from build123d import *

# Parameters (mm, degrees)
SKETCH_1_W          = 125.6
SKETCH_1_H          = 165
SKETCH_1_R          = 2
SKETCH_1_R_2        = 12.5
SKETCH_1_R_3        = 2.25
SKETCH_1_R_4        = 1.5
SKETCH_1_W_2        = 10
SKETCH_1_H_2        = 23
SKETCH_1_W_3        = 16
SKETCH_1_H_3        = 40
EXTRUDE_1_DEPTH     = 1.5
SKETCH_2_W          = 1.2
SKETCH_2_H          = 100
SKETCH_2_H_2        = 50
EXTRUDE_2_DEPTH     = 45
SKETCH_3_W          = 125.6
SKETCH_3_H          = 1.2
SKETCH_3_W_2        = 22.4
EXTRUDE_3_DEPTH     = 5
SKETCH_4_W          = 22.4
SKETCH_4_H          = 3
SKETCH_4_W_2        = 125.6
EXTRUDE_4_DEPTH     = 1
SKETCH_5_W          = 125.6
SKETCH_5_H          = 3
EXTRUDE_5_DEPTH     = 1
FILLET_1_R          = 40
SKETCH_6_R          = 1.5
EXTRUDE_6_DEPTH     = 2
EXTRUDE_7_DEPTH     = 30
CUT_EXTRUDE_1_REACH = 214.515
SKETCH_9_R          = 1.5
SKETCH_10_R         = 1.5
CUT_EXTRUDE_2_DEPTH = 213.514964179
SKETCH_11_R         = 1.5
CUT_EXTRUDE_3_DEPTH = 213.514964179


with BuildPart() as part:
    # 草图1 → 凸台-拉伸1 (new body)
    with BuildSketch(Plane(origin=(0, 0, 0), x_dir=(1, 0, 0), z_dir=(0, 1, 0))):
        with Locations((62.8, 82.5)):
            Rectangle(SKETCH_1_W, SKETCH_1_H)
        with Locations(Location((93.2, 30, 0), (0, 0, 270))):
            Circle(SKETCH_1_R, mode=Mode.SUBTRACT)
        with Locations(Location((93.2, 88, 0), (0, 0, 270))):
            Circle(SKETCH_1_R, mode=Mode.SUBTRACT)
        with Locations(Location((7.2, 30, 0), (0, 0, 90))):
            Circle(SKETCH_1_R, mode=Mode.SUBTRACT)
        with Locations(Location((7.2, 88, 0), (0, 0, 90))):
            Circle(SKETCH_1_R, mode=Mode.SUBTRACT)
        with Locations(Location((33.8, 135, 0), (0, 0, 270))):
            Circle(SKETCH_1_R_2, mode=Mode.SUBTRACT)
        with Locations(Location((91.8, 135, 0), (0, 0, 90))):
            Circle(SKETCH_1_R_2, mode=Mode.SUBTRACT)
        with Locations(Location((49.3, 150.5, 0), (0, 0, 270))):
            Circle(SKETCH_1_R_3, mode=Mode.SUBTRACT)
        with Locations(Location((18.3, 150.5, 0), (0, 0, 90))):
            Circle(SKETCH_1_R_3, mode=Mode.SUBTRACT)
        with Locations(Location((49.3, 119.5, 0), (0, 0, 90))):
            Circle(SKETCH_1_R_3, mode=Mode.SUBTRACT)
        with Locations(Location((18.3, 119.5, 0), (0, 0, 270))):
            Circle(SKETCH_1_R_3, mode=Mode.SUBTRACT)
        with Locations(Location((107.3, 119.5, 0), (0, 0, 90))):
            Circle(SKETCH_1_R_3, mode=Mode.SUBTRACT)
        with Locations(Location((76.3, 119.5, 0), (0, 0, 270))):
            Circle(SKETCH_1_R_3, mode=Mode.SUBTRACT)
        with Locations(Location((107.3, 150.5, 0), (0, 0, 270))):
            Circle(SKETCH_1_R_3, mode=Mode.SUBTRACT)
        with Locations(Location((76.3, 150.5, 0), (0, 0, 90))):
            Circle(SKETCH_1_R_3, mode=Mode.SUBTRACT)
        with Locations(Location((122.1, 161, 0), (0, 0, 270))):
            Circle(SKETCH_1_R_4, mode=Mode.SUBTRACT)
        with Locations(Location((122.1, 109, 0), (0, 0, 90))):
            Circle(SKETCH_1_R_4, mode=Mode.SUBTRACT)
        with Locations(Location((109.1, 109, 0), (0, 0, 270))):
            Circle(SKETCH_1_R_4, mode=Mode.SUBTRACT)
        with Locations(Location((109.1, 161, 0), (0, 0, 90))):
            Circle(SKETCH_1_R_4, mode=Mode.SUBTRACT)
        with Locations(Location((16.5, 109, 0), (0, 0, 90))):
            Circle(SKETCH_1_R_4, mode=Mode.SUBTRACT)
        with Locations(Location((3.5, 109, 0), (0, 0, 270))):
            Circle(SKETCH_1_R_4, mode=Mode.SUBTRACT)
        with Locations(Location((16.5, 161, 0), (0, 0, 270))):
            Circle(SKETCH_1_R_4, mode=Mode.SUBTRACT)
        with Locations(Location((3.5, 161, 0), (0, 0, 90))):
            Circle(SKETCH_1_R_4, mode=Mode.SUBTRACT)
        with Locations(Location((69.1, 109, 0), (0, 0, 270))):
            Circle(SKETCH_1_R_4, mode=Mode.SUBTRACT)
        with Locations(Location((82.1, 109, 0), (0, 0, 90))):
            Circle(SKETCH_1_R_4, mode=Mode.SUBTRACT)
        with Locations(Location((82.1, 161, 0), (0, 0, 270))):
            Circle(SKETCH_1_R_4, mode=Mode.SUBTRACT)
        with Locations(Location((69.1, 161, 0), (0, 0, 90))):
            Circle(SKETCH_1_R_4, mode=Mode.SUBTRACT)
        with Locations(Location((56.5, 161, 0), (0, 0, 270))):
            Circle(SKETCH_1_R_4, mode=Mode.SUBTRACT)
        with Locations(Location((43.5, 161, 0), (0, 0, 90))):
            Circle(SKETCH_1_R_4, mode=Mode.SUBTRACT)
        with Locations(Location((56.5, 109, 0), (0, 0, 90))):
            Circle(SKETCH_1_R_4, mode=Mode.SUBTRACT)
        with Locations(Location((43.5, 109, 0), (0, 0, 270))):
            Circle(SKETCH_1_R_4, mode=Mode.SUBTRACT)
        with Locations(Location((4, 100, 0), (0, 0, 270))):
            Circle(SKETCH_1_R_4, mode=Mode.SUBTRACT)
        with Locations(Location((4, 6, 0), (0, 0, 270))):
            Circle(SKETCH_1_R_4, mode=Mode.SUBTRACT)
        with Locations(Location((121.6, 6, 0), (0, 0, 90))):
            Circle(SKETCH_1_R_4, mode=Mode.SUBTRACT)
        with Locations(Location((121.6, 100, 0), (0, 0, 90))):
            Circle(SKETCH_1_R_4, mode=Mode.SUBTRACT)
        with Locations((114.4, 66.5)):
            Rectangle(SKETCH_1_W_2, SKETCH_1_H_2, mode=Mode.SUBTRACT)
        with Locations((62.8, 135)):
            Rectangle(SKETCH_1_W_3, SKETCH_1_H_3, mode=Mode.SUBTRACT)
    extrude(amount=EXTRUDE_1_DEPTH)

    # 草图2 → 凸台-拉伸2 (add)
    with BuildSketch(Plane(origin=(0, 1.5, 0), x_dir=(1, 0, 0), z_dir=(0, 1, 0))):
        with Locations((0.6, 50)):
            Rectangle(SKETCH_2_W, SKETCH_2_H)
        with Locations((103.8, 25)):
            Rectangle(SKETCH_2_W, SKETCH_2_H_2)
        with Locations((125, 50)):
            Rectangle(SKETCH_2_W, SKETCH_2_H)
    extrude(amount=EXTRUDE_2_DEPTH)

    # 草图3 → 凸台-拉伸3 (add)
    with BuildSketch(Plane(origin=(0, 1.5, 0), x_dir=(1, 0, 0), z_dir=(0, 1, 0))):
        with Locations((62.8, 0.6)):
            Rectangle(SKETCH_3_W, SKETCH_3_H)
        with Locations((62.8, 99.4)):
            Rectangle(SKETCH_3_W, SKETCH_3_H)
        with Locations((114.4, 47.8)):
            Rectangle(SKETCH_3_W_2, SKETCH_3_H)
    extrude(amount=EXTRUDE_3_DEPTH)

    # 草图4 → 凸台-拉伸4 (add)
    with BuildSketch(Plane.XY):
        with Locations((114.4, 23.5)):
            Rectangle(SKETCH_4_W, SKETCH_4_H)
        with Locations((62.8, 44.7)):
            Rectangle(SKETCH_4_W_2, SKETCH_4_H)
    extrude(amount=-EXTRUDE_4_DEPTH)

    # 草图5 → 凸台-拉伸5 (add)
    with BuildSketch(Plane(origin=(0, 0, -100), x_dir=(-1, 0, 0), z_dir=(0, 0, -1))):
        with Locations((-62.8, 44.7)):
            Rectangle(SKETCH_5_W, SKETCH_5_H)
    extrude(amount=-EXTRUDE_5_DEPTH)

    # 圆角1
    fillet_1_edges = [part.edges().sort_by_distance(p)[0] for p in [
        (103.8, 46.5, -50),
    ]]
    fillet(fillet_1_edges, radius=FILLET_1_R)

    # 草图6 → 凸台-拉伸6 (add)
    # profile 1 of 4: a face of its own
    with BuildSketch(Plane(origin=(0, 46.5, 0), x_dir=(1, 0, 0), z_dir=(0, 1, 0))):
        with BuildLine():
            Line((0, 0), (10, 0))
            Line((10, 0), (10, 7))
            ThreePointArc((10, 7), (9.121320344, 9.121320344), (7, 10))
            Line((7, 10), (0, 10))
            Line((0, 10), (0, 0))
        make_face()
        with Locations(Location((5, 5, 0), (0, 0, 270))):
            Circle(SKETCH_6_R, mode=Mode.SUBTRACT)
    # profile 2 of 4: a face of its own
    with BuildSketch(Plane(origin=(0, 46.5, 0), x_dir=(1, 0, 0), z_dir=(0, 1, 0))):
        with BuildLine():
            Line((10, 100), (10, 93))
            ThreePointArc((10, 93), (9.121320344, 90.878679656), (7, 90))
            Line((7, 90), (0, 90))
            Line((0, 90), (0, 100))
            Line((0, 100), (10, 100))
        make_face()
        with Locations(Location((5, 95, 0), (0, 0, 90))):
            Circle(SKETCH_6_R, mode=Mode.SUBTRACT)
    # profile 3 of 4: a face of its own
    with BuildSketch(Plane(origin=(0, 46.5, 0), x_dir=(1, 0, 0), z_dir=(0, 1, 0))):
        with BuildLine():
            Line((94.4, 0), (94.4, 7))
            ThreePointArc((94.4, 7), (95.278679656, 9.121320344), (97.4, 10))
            Line((97.4, 10), (104.4, 10))
            Line((104.4, 10), (104.4, 0))
            Line((104.4, 0), (94.4, 0))
        make_face()
        with Locations(Location((99.4, 5, 0), (0, 0, 90))):
            Circle(SKETCH_6_R, mode=Mode.SUBTRACT)
    # profile 4 of 4: a face of its own
    with BuildSketch(Plane(origin=(0, 46.5, 0), x_dir=(1, 0, 0), z_dir=(0, 1, 0))):
        with BuildLine():
            Line((125.6, 100), (115.6, 100))
            Line((115.6, 100), (115.6, 93))
            ThreePointArc((115.6, 93), (116.478679656, 90.878679656), (118.6, 90))
            Line((118.6, 90), (125.6, 90))
            Line((125.6, 90), (125.6, 100))
        make_face()
        with Locations(Location((120.6, 95, 0), (0, 0, 270))):
            Circle(SKETCH_6_R, mode=Mode.SUBTRACT)
    extrude(amount=-EXTRUDE_6_DEPTH)

    # 草图8 → 凸台-拉伸7 (add)
    with BuildSketch(Plane(origin=(0, 1.5, 0), x_dir=(1, 0, 0), z_dir=(0, 1, 0))):
        Polygon((125.6, 100), (124.6, 100), (124.6, 163.8), (1, 163.8), (1, 100), (0, 100), (0, 165), (125.6, 165), align=None)
    extrude(amount=EXTRUDE_7_DEPTH)

    # 草图9 → 切除-拉伸1 (cut, up to next)
    with BuildSketch(Plane(origin=(0, 0, -165), x_dir=(-1, 0, 0), z_dir=(0, 0, -1)), mode=Mode.PRIVATE) as cut_extrude_1_sk1:
        with Locations((-33.8, 26.5)):
            Circle(SKETCH_9_R)
    cut_extrude_1_tool1 = extrude(cut_extrude_1_sk1.sketch, amount=-CUT_EXTRUDE_1_REACH, mode=Mode.PRIVATE) & part.part
    # 草图9 → 切除-拉伸1 (cut, up to next)
    with BuildSketch(Plane(origin=(0, 0, -165), x_dir=(-1, 0, 0), z_dir=(0, 0, -1)), mode=Mode.PRIVATE) as cut_extrude_1_sk2:
        with Locations((-21.8, 26.5)):
            Circle(SKETCH_9_R)
    cut_extrude_1_tool2 = extrude(cut_extrude_1_sk2.sketch, amount=-CUT_EXTRUDE_1_REACH, mode=Mode.PRIVATE) & part.part
    # 草图9 → 切除-拉伸1 (cut, up to next)
    with BuildSketch(Plane(origin=(0, 0, -165), x_dir=(-1, 0, 0), z_dir=(0, 0, -1)), mode=Mode.PRIVATE) as cut_extrude_1_sk3:
        with Locations((-21.8, 11.5)):
            Circle(SKETCH_9_R)
    cut_extrude_1_tool3 = extrude(cut_extrude_1_sk3.sketch, amount=-CUT_EXTRUDE_1_REACH, mode=Mode.PRIVATE) & part.part
    # 草图9 → 切除-拉伸1 (cut, up to next)
    with BuildSketch(Plane(origin=(0, 0, -165), x_dir=(-1, 0, 0), z_dir=(0, 0, -1)), mode=Mode.PRIVATE) as cut_extrude_1_sk4:
        with Locations((-33.8, 11.5)):
            Circle(SKETCH_9_R)
    cut_extrude_1_tool4 = extrude(cut_extrude_1_sk4.sketch, amount=-CUT_EXTRUDE_1_REACH, mode=Mode.PRIVATE) & part.part
    # 草图9 → 切除-拉伸1 (cut, up to next)
    with BuildSketch(Plane(origin=(0, 0, -165), x_dir=(-1, 0, 0), z_dir=(0, 0, -1)), mode=Mode.PRIVATE) as cut_extrude_1_sk5:
        with Locations((-81.3, 11.5)):
            Circle(SKETCH_9_R)
    cut_extrude_1_tool5 = extrude(cut_extrude_1_sk5.sketch, amount=-CUT_EXTRUDE_1_REACH, mode=Mode.PRIVATE) & part.part
    # 草图9 → 切除-拉伸1 (cut, up to next)
    with BuildSketch(Plane(origin=(0, 0, -165), x_dir=(-1, 0, 0), z_dir=(0, 0, -1)), mode=Mode.PRIVATE) as cut_extrude_1_sk6:
        with Locations((-93.3, 11.5)):
            Circle(SKETCH_9_R)
    cut_extrude_1_tool6 = extrude(cut_extrude_1_sk6.sketch, amount=-CUT_EXTRUDE_1_REACH, mode=Mode.PRIVATE) & part.part
    # 草图9 → 切除-拉伸1 (cut, up to next)
    with BuildSketch(Plane(origin=(0, 0, -165), x_dir=(-1, 0, 0), z_dir=(0, 0, -1)), mode=Mode.PRIVATE) as cut_extrude_1_sk7:
        with Locations((-93.3, 26.5)):
            Circle(SKETCH_9_R)
    cut_extrude_1_tool7 = extrude(cut_extrude_1_sk7.sketch, amount=-CUT_EXTRUDE_1_REACH, mode=Mode.PRIVATE) & part.part
    # 草图9 → 切除-拉伸1 (cut, up to next)
    with BuildSketch(Plane(origin=(0, 0, -165), x_dir=(-1, 0, 0), z_dir=(0, 0, -1)), mode=Mode.PRIVATE) as cut_extrude_1_sk8:
        with Locations((-81.3, 26.5)):
            Circle(SKETCH_9_R)
    cut_extrude_1_tool8 = extrude(cut_extrude_1_sk8.sketch, amount=-CUT_EXTRUDE_1_REACH, mode=Mode.PRIVATE) & part.part
    add(cut_extrude_1_tool1.solids().sort_by_distance((33.8, 26.5, -165))[0], mode=Mode.SUBTRACT)
    add(cut_extrude_1_tool2.solids().sort_by_distance((21.8, 26.5, -165))[0], mode=Mode.SUBTRACT)
    add(cut_extrude_1_tool3.solids().sort_by_distance((21.8, 11.5, -165))[0], mode=Mode.SUBTRACT)
    add(cut_extrude_1_tool4.solids().sort_by_distance((33.8, 11.5, -165))[0], mode=Mode.SUBTRACT)
    add(cut_extrude_1_tool5.solids().sort_by_distance((81.3, 11.5, -165))[0], mode=Mode.SUBTRACT)
    add(cut_extrude_1_tool6.solids().sort_by_distance((93.3, 11.5, -165))[0], mode=Mode.SUBTRACT)
    add(cut_extrude_1_tool7.solids().sort_by_distance((93.3, 26.5, -165))[0], mode=Mode.SUBTRACT)
    add(cut_extrude_1_tool8.solids().sort_by_distance((81.3, 26.5, -165))[0], mode=Mode.SUBTRACT)

    # 草图10 → 切除-拉伸2 (cut, through all)
    with BuildSketch(Plane(origin=(125.6, 0, 0), x_dir=(0, 0, -1), z_dir=(1, 0, 0))):
        with Locations((96, 42.5)):
            Circle(SKETCH_10_R)
        with Locations((6, 42.5)):
            Circle(SKETCH_10_R)
    extrude(amount=-CUT_EXTRUDE_2_DEPTH, mode=Mode.SUBTRACT)

    # 草图11 → 切除-拉伸3 (cut, through all)
    with BuildSketch(Plane(origin=(125.6, 0, 0), x_dir=(0, 0, -1), z_dir=(1, 0, 0))):
        with Locations((160, 26.5)):
            Circle(SKETCH_11_R)
        with Locations((106, 26.5)):
            Circle(SKETCH_11_R)
    extrude(amount=-CUT_EXTRUDE_3_DEPTH, mode=Mode.SUBTRACT)


solid = part.part
Design review of the part built by this model. Coordinates are the model's own, in mm. A direction names the side the tool comes from. Give positions to 0.01 mm unless a question says otherwise; leave off trailing zeros. Write each loop counter-clockwise with the first axis right and the second up, starting at its lowest first coordinate (ties: lowest second). Pieces come first, ordered by that corner, then holes. Notation, with made-up numbers: M 33.25,79.5 L 69.25,79.5 A23 cw 69.25,89.5 Z; hole C 50.5,4.5 d3. An arc over 180 degrees is marked long. Answer as a JSON object with one key per item and string values. Group by question number.
1) We need section C-C (x = 49.3). Give the boundary of the cut face in (y, z).
2) We need section B-B (z = -134.5). Give the boundary of the cut face in (x, y), and give its area (3 significant figures).
3) Clearance check with flat-ended pins moving along their axes: pin 1 Ø0.6 at (x, z) = (122, -99.5) entering from -Y; pin 2 Ø2 at (y, z) = (17, -93) entering from -X; pin 3 Ø1.8 at (x, y) = (81.3, 26.5) entering from -Z; pin 4 Ø1.3 at (x, z) = (112, -0.5) entering from +Y. State where each tip first meets the part, or that it passes through.
4) Mouldability with a two-part tool opening along X and no side actions: class faces 1 (the face through (125.6, 18, -84)), 2 (the face through (104.4, 24, -25)), 3 (the face through (7.966, 0.74, -31.847)), 4 (the face through (98, 46.5, -4)) as released by +X, released by -X, zero draft, split by the parting line, or undercut.
5) We need section D-D (z = -75). Give the boundary of the cut face in (x, y).
6) For line 1 along Z through (x, y) = (99.4, 45.35); line 2 along X through (y, z) = (31, -29.5); line 3 along Z through (x, y) = (91, 4.5), list the stretches that pass through material, from the lowest coordinate up.
7) We need section A-A (y = 4.5). Give the boundary of the cut face in (x, z), and give its area (3 significant figures).
8) Tool access review of faces 5 (the face through (105.403, 0.74, -120.71)), 6 (the face through (114, 4, -47.2)), 7 (the face through (51, 4, -1.2)): name each direction out of +Z, -Z, +X, -X, +Y, -Y from which nothing blocks a thin tool from reaching the whole face with its end or side.
Answer key:
{
 "1": {"outline": "M 0,-165 L 31.5,-165 L 31.5,-163.8 L 1.5,-163.8 L 1.5,-152.75 L 0,-152.75 Z; M 0,-148.25 L 1.5,-148.25 L 1.5,-121.75 L 0,-121.75 Z; M 0,-117.25 L 1.5,-117.25 L 1.5,-100 L 6.5,-100 L 6.5,-98.8 L 1.5,-98.8 L 1.5,-1.2 L 6.5,-1.2 L 6.5,0 L 0,0 Z; M 43.2,-100 L 46.2,-100 L 46.2,-99 L 43.2,-99 Z; M 43.2,-1 L 46.2,-1 L 46.2,0 L 43.2,0 Z"},
 "2": {"outline": "M 0,0 L 21.31,0 L 21.31,1.5 L 1,1.5 L 1,31.5 L 0,31.5 Z; M 46.29,0 L 54.8,0 L 54.8,1.5 L 46.29,1.5 Z; M 70.8,0 L 79.31,0 L 79.31,1.5 L 70.8,1.5 Z; M 104.29,0 L 125.6,0 L 125.6,31.5 L 124.6,31.5 L 124.6,1.5 L 104.29,1.5 Z", "area": "149 mm²"},
 "3": {"pin 1": "stops at y = 1.5", "pin 2": "stops at x = 0", "pin 3": "passes through", "pin 4": "stops at y = 46.2"},
 "4": {"face 1": "released by +X", "face 2": "undercut", "face 3": "undercut", "face 4": "zero draft"},
 "5": {"outline": "M 0,0 L 109.4,0 L 109.4,1.5 L 1.2,1.5 L 1.2,46.5 L 0,46.5 Z; M 119.4,0 L 125.6,0 L 125.6,46.5 L 124.4,46.5 L 124.4,1.5 L 119.4,1.5 Z"},
 "6": {"line 1": "z = -100 to -99, -10 to -6.5, -3.5 to 0", "line 2": "x = 0 to 1.2, 103.2 to 104.4, 124.4 to 125.6", "line 3": "z = -165 to -163.8, -100 to -98.8, -1.2 to 0"},
 "7": {"outline": "M 0,-165 L 125.6,-165 L 125.6,0 L 0,0 Z; hole M 1,-163.8 L 124.6,-163.8 L 124.6,-100 L 1,-100 Z; hole M 1.2,-98.8 L 124.4,-98.8 L 124.4,-48.4 L 104.4,-48.4 L 104.4,-50 L 103.2,-50 L 103.2,-1.2 L 1.2,-1.2 Z; hole M 104.4,-47.2 L 124.4,-47.2 L 124.4,-1.2 L 104.4,-1.2 Z", "area": "897 mm²"},
 "8": {"face 5": "+Y, -Y", "face 6": "+Y", "face 7": "none"}
}
